Work out the finished part from the listing and answer in its coordinate system (mm). A direction names the side the tool comes from. Coordinates: 2 decimals unless noted, no trailing zeros. Loops run counter-clockwise (first coordinate to the right, second up) from the corner with the lowest first, then second, coordinate; pieces in that order, holes last. Notation, with made-up numbers: (-39.5, 32.5) -> (11.5, 32.5) arc R4 cw to (11.5, 38.5) -> close; hole circle Ø6 at (47, 63.5). An arc over 180 degrees is marked (long way). Use a Markdown table: item, result.
from build123d import *

# Parameters (mm, degrees)
F0_W     = 50
F0_H     = 50
F1_DEPTH = 50
F2_R     = 20
F3_T     = -2.5


with BuildPart() as f1:
    # F0 (on Top) → F1 (new body)
    with BuildSketch(Plane.XY):
        with Locations((0, 1.597746)):
            Rectangle(F0_W, F0_H)
    extrude(amount=F1_DEPTH)

    # F2
    f2_edges = [f1.edges().sort_by_distance(p)[0] for p in [
        (25, 1.597746, 0),
        (-25, 1.597746, 0),
        (25, 1.597746, 50),
        (-25, 1.597746, 50),
    ]]
    fillet(f2_edges, radius=F2_R)

    # F3
    f3_openings = [f1.faces().sort_by_distance(p)[0] for p in [
        (0, -23.402254, 25),
    ]]
    offset(amount=F3_T, openings=f3_openings)


solid = f1.part
Q1. Given pin 1 Ø6 at (x, y) = (-16, 8.5) entering from +Z; pin 2 Ø5 at (y, z) = (9, 38.5) entering from -X; pin 3 Ø12 at (y, z) = (-16.5, 8.5) entering from +X, each flat-ended and moving along its own axis, determine where each tip first touches the part or whether it passes through.
Solved:
| item | result |
|---|---|
| pin 1 | z = 48.33 |
| pin 2 | x = -24.08 |
| pin 3 | x = 24.23 |
Q2. Section A-A on y = -18 is taken. Determine the outline of the cut face in (x, z).
Solved:
| item | result |
|---|---|
| outline | (-25, 20) arc R20 ccw to (-5, 0) -> (5, 0) arc R20 ccw to (25, 20) -> (25, 30) arc R20 ccw to (5, 50) -> (-5, 50) arc R20 ccw to (-25, 30) -> close; hole (-22.5, 20) arc R17.5 ccw to (-5, 2.5) -> (5, 2.5) arc R17.5 ccw to (22.5, 20) -> (22.5, 30) arc R17.5 ccw to (5, 47.5) -> (-5, 47.5) arc R17.5 ccw to (-22.5, 30) -> close |
Q3. For faces 1 (the cylindrical face through (17.51, 0.68, 7.76)), 2 (the cylindrical face through (19.297, 1.948, 43.986)), determine the directions among +Z, -Z, +X, -X, +Y, -Y from which every point of the face is accessible in a straight line to the end or side of a thin tool.
Solved:
| item | result |
|---|---|
| face 1 | -Y |
| face 2 | +Z, +X, +Y, -Y |
Q4. Section B-B on x = -3 is taken. Determine the outline of the cut face in (y, z).
Solved:
| item | result |
|---|---|
| outline | (-23.4, 0) -> (26.6, 0) -> (26.6, 50) -> (-23.4, 50) -> (-23.4, 47.5) -> (24.1, 47.5) -> (24.1, 2.5) -> (-23.4, 2.5) -> close |
Q5. Consider line 1 (X direction, y = 12, z = 21); line 2 (Z direction, x = -5, y = 1); line 3 (X direction, y = -12.5, z = 15.5). Determine where each line is inside the solid, lowest interval first. Write a range as [from, to].
Solved:
| item | result |
|---|---|
| line 1 | [-25, -22.5], [22.5, 25] |
| line 2 | [0, 2.5], [47.5, 50] |
| line 3 | [-24.49, -21.91], [21.91, 24.49] |
Q6. Section C-C on z = 22 is taken. Determine the outline of the cut face in (x, y), and give its area (4 significant figures).
Solved:
| item | result |
|---|---|
| outline | (-25, -23.4) -> (-22.5, -23.4) -> (-22.5, 24.1) -> (22.5, 24.1) -> (22.5, -23.4) -> (25, -23.4) -> (25, 26.6) -> (-25, 26.6) -> close |
| area | 362.5 mm² |
Q7. Determine the mould class of faces 3 (the flat face through (25, 1, 25)), 4 (the flat face through (0, 26.598, 25)), 5 (the flat face through (0, 1, 47.5)) for opening direction X: pulls with the +X half, pulls with the -X half, needs draft (parallel to the pull), parting line crosses it, or undercut.
Solved:
| item | result |
|---|---|
| face 3 | pulls with the +X half |
| face 4 | needs draft |
| face 5 | undercut |
